```python
from build123d import *

# Parameters (mm, degrees)
SKETCH_1_R          = 2.1
EXTRUDE_1_DEPTH     = 11
EXTRUDE_2_DEPTH     = 79
SKETCH_3_R          = 2.1
EXTRUDE_3_DEPTH     = 10
EXTRUDE_START       = -10
SKETCH_3_2_R        = 2.1
EXTRUDE_4_DEPTH     = 10
CUT_EXTRUDE_6_DEPTH = 10


with BuildPart() as part:
    # Sketch 1 → Extrude 1 (new body)
    with BuildSketch(Plane(origin=(0, 139.195974268, 0), x_dir=(1, 0, 0), z_dir=(0, 1, 0))):
        Polygon((21.558980694, -32.273129836), (1.558980694, -32.273129836), (1.558980694, -68.304125072), (6.558980694, -68.273129836), (6.558980694, -56.273129836), (21.558980694, -56.273129836), align=None)
        with Locations(Location((11.55898069, -40.273129836, 0), (0, 0, 180))):
            Circle(SKETCH_1_R, mode=Mode.SUBTRACT)
    extrude(amount=EXTRUDE_1_DEPTH)

    # Sketch 2 → Extrude 2 (add)
    with BuildSketch(Plane(origin=(0, 150.195974268, 0), x_dir=(1, 0, 0), z_dir=(0, 1, 0))):
        Polygon((1.558980694, -32.273129836), (4.558980694, -32.273129836), (4.558980694, -48.273129836), (21.558980694, -48.273129836), (21.558980694, -56.273129836), (9.808980694, -56.273129836), (9.808980694, -103.773129836), (2.558980694, -110.773129836), (1.558980694, -110.773129836), align=None)
    extrude(amount=EXTRUDE_2_DEPTH)



with BuildPart() as body_2:
    # Sketch 3 → Extrude 3 (new body)
    with BuildSketch(Plane(origin=(0, 239.195974268, 0), x_dir=(1, 0, 0), z_dir=(0, 1, 0))):
        Polygon((1.558980694, -32.273129836), (1.558980694, -110.773129836), (2.558980694, -110.773129836), (9.808980694, -103.773129836), (9.808980694, -56.273129836), (21.558980694, -56.273129836), (21.558980694, -32.273129836), align=None)
        with Locations(Location((11.55898069, -40.273129836, 0), (0, 0, 180))):
            Circle(SKETCH_3_R, mode=Mode.SUBTRACT)
    extrude(amount=EXTRUDE_3_DEPTH)


with BuildPart() as part_1:
    add(part.part)

    add(body_2.part)  # Extrude 4 merges body 2
    # Sketch 3_2 → Extrude 4 (add)
    with BuildSketch(Plane(origin=(0, 239.195974268, 0), x_dir=(1, 0, 0), z_dir=(0, 1, 0)).offset(EXTRUDE_START)):
        Polygon((1.558980694, -32.273129836), (1.558980694, -110.773129836), (2.558980694, -110.773129836), (9.808980694, -103.773129836), (9.808980694, -56.273129836), (21.558980694, -56.273129836), (21.558980694, -32.273129836), align=None)
        with Locations(Location((11.55898069, -40.273129836, 0), (0, 0, 180))):
            Circle(SKETCH_3_2_R, mode=Mode.SUBTRACT)
    extrude(amount=EXTRUDE_4_DEPTH)

    # Sketch 5 → Cut-Extrude 6 (cut)
    with BuildSketch(Plane(origin=(0, 249.195974268, 0), x_dir=(1, 0, 0), z_dir=(0, 1, 0))):
        Polygon((1.558980694, -110.773129836), (1.558980694, -48.273129836), (21.558980694, -48.273129836), (21.558980694, -56.273129836), (9.808980694, -56.273129836), (9.808980694, -103.773129836), (2.558980694, -110.773129836), align=None)
    extrude(amount=-CUT_EXTRUDE_6_DEPTH, mode=Mode.SUBTRACT)


solid = part_1.part
```
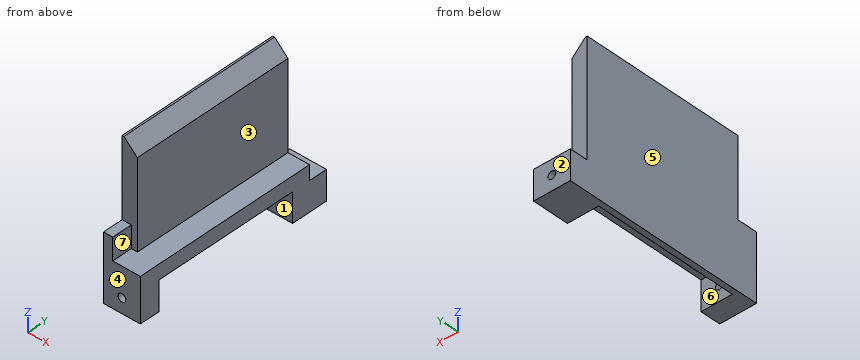
Input: part model. Units: mm. Frame: model coordinates. Face numbers are marked on the shaded views. A direction names the side the tool comes from. Give positions to 0.01 mm unless a question says otherwise; leave off trailing zeros. Loops run counter-clockwise (first coordinate to the right, second up) from the corner with the lowest first, then second, coordinate; pieces in that order, holes last. Notation, with made-up numbers: (51, -40) -> (87, -40) arc R31 ccw to (87, -6) -> close; hole circle Ø2 at (4.5, 68.25). An arc over 180 degrees is marked (long way). Use a Markdown table: item, result.
Q1. Section query C-C, the plane z = 65. Return the cut outline in (x, y), plus the area to 3 significant figures.
Entries:
| item | result |
|---|---|
| outline | (1.56, 139.2) -> (6.56, 139.2) -> (6.56, 150.2) -> (9.81, 150.2) -> (9.81, 239.2) -> (1.56, 239.2) -> close |
| area | 789 mm² |
Q2. Access query for the marked faces 5, 6 and 7. Directions: +Z, -Z, +X, -X, +Y, -Y. A direction counts if a zero-diameter tool reaches every point of the face in a straight line with its end or side. Return the directions, or none.
Entries:
| item | result |
|---|---|
| face 5 | +Z, -Z, -X, +Y, -Y |
| face 6 | -Z, +X |
| face 7 | +Z, +X, -Y |
Q3. Section query D-D, the plane x = 7.75. Return the cut outline in (y, z).
Entries:
| item | result |
|---|---|
| outline | (139.2, 32.27) -> (150.2, 32.27) -> (150.2, 48.27) -> (229.2, 48.27) -> (229.2, 32.27) -> (249.2, 32.27) -> (249.2, 48.27) -> (239.2, 48.27) -> (239.2, 105.76) -> (150.2, 105.76) -> (150.2, 56.27) -> (139.2, 56.27) -> close |
Q4. First-contact query: P1, Ø3.5, axis at x = 11.56, z = 40.27, coming from the -Y side (1 decimal); P2, Ø10, axis at x = 16, y = 161, coming from the +Z side; P3, Ø5, axis at x = 9.5, y = 246.5, coming from the +Z side; P4, Ø1, axis at x = 10, y = 222.5, coming from the -Z side. Flat tips, straight axial feed; report the tip coordinate or a pass-through.
Entries:
| item | result |
|---|---|
| P1 | passes through |
| P2 | stops at z = 56.27 |
| P3 | stops at z = 48.27 |
| P4 | stops at z = 48.27 |
Q5. Section query B-B, the plane y = 172. Return the cut outline in (x, z).
Entries:
| item | result |
|---|---|
| outline | (1.56, 32.27) -> (4.56, 32.27) -> (4.56, 48.27) -> (21.56, 48.27) -> (21.56, 56.27) -> (9.81, 56.27) -> (9.81, 103.77) -> (2.56, 110.77) -> (1.56, 110.77) -> close |
Q6. Section query A-A, the plane x = 17. Return the cut outline in (y, z).
Entries:
| item | result |
|---|---|
| outline | (139.2, 32.27) -> (150.2, 32.27) -> (150.2, 48.27) -> (229.2, 48.27) -> (229.2, 32.27) -> (249.2, 32.27) -> (249.2, 48.27) -> (239.2, 48.27) -> (239.2, 56.27) -> (139.2, 56.27) -> close |
Q7. Ray query, probe 1 along Y at (x, z) = (19.5, 42); probe 2 along Y at (x, z) = (5.75, 95.5); probe 3 along Z at (x, y) = (12.25, 156.5). Return the intervals inside material, ascending. Write a range as from..to.
Entries:
| item | result |
|---|---|
| probe 1 | y = 139.2..150.2, 229.2..249.2 |
| probe 2 | y = 150.2..239.2 |
| probe 3 | z = 48.27..56.27 |
Q8. Pull-direction query (Y, two-part tool) for the marked faces 1, 2, 3 and 4; classes: pulls with the +Y half, pulls with the -Y half, needs draft (parallel to the pull), parting line crosses it, or undercut.
Entries:
| item | result |
|---|---|
| face 1 | undercut |
| face 2 | pulls with the +Y half |
| face 3 | needs draft |
| face 4 | pulls with the -Y half |
